Design review of the part shown in the three views and the two pictorial views. Dimensions are in mm from the part's minimum x, y and z. Coordinates: 2 decimals unless noted, no trailing zeros. Loops run counter-clockwise (first coordinate to the right, second up) from the corner with the lowest first, then second, coordinate; pieces in that order, holes last. Notation, with made-up numbers: (-7, 81.25) -> (31, 81.25) arc R25 cw to (31, 117.25) -> close; hole circle Ø8 at (-33, 60). An arc over 180 degrees is marked (long way). One line per item, written item: value.
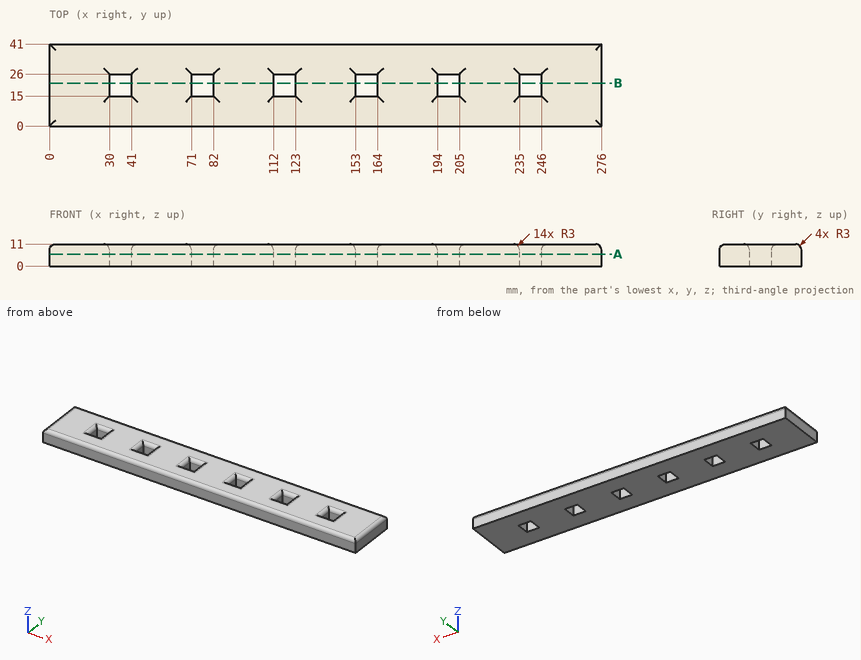
1. Take a section at B-B, the plane y = 21.5. Give the number of separate pieces and of enclosed holes in the cut face, and give its area (3 significant figures).
Return value:
separate pieces: 7
enclosed holes: 0
area: 2,280 mm2
2. Take a section at A-A, the plane z = 6. Give the boundary of the cut face in (x, y).
Return value:
outline: (0, 0) -> (276, 0) -> (276, 41) -> (0, 41) -> close; hole (30, 15) -> (41, 15) -> (41, 26) -> (30, 26) -> close; hole (71, 15) -> (82, 15) -> (82, 26) -> (71, 26) -> close; hole (112, 15) -> (123, 15) -> (123, 26) -> (112, 26) -> close; hole (153, 15) -> (164, 15) -> (164, 26) -> (153, 26) -> close; hole (194, 15) -> (205, 15) -> (205, 26) -> (194, 26) -> close; hole (235, 15) -> (246, 15) -> (246, 26) -> (235, 26) -> close
3. To check wall thickness, follow probe 1 along Y at (x, z) = (122, 6.5); probe 2 along X at (y, z) = (39.5, 8.25); probe 3 along Y at (x, z) = (79.5, 9.5). State the ranges of each line that lie inside material, in increasing order. Write a range as from..to.
Return value:
probe 1: y = 0..15, 26..41
probe 2: x = 0.01..275.99
probe 3: y = 0.4..14.6, 26.4..40.6
